Autodesk Inventor part; units mm, degrees
ref_plane "YZ Plane" through (0, 0, 0) normal (1, 0, 0) x (0, 1, 0)
ref_plane "XZ Plane" through (0, 0, 0) normal (0, 1, 0) x (-1, 0, 0)
ref_plane "XY Plane" through (0, 0, 0) normal (0, 0, 1) x (1, 0, 0)
sketch "Sketch1" plane through (0, 0, 0) normal (0, 0, 1) x (1, 0, 0)
  arc A0 (0, 0) -> (0.159434, 1.869277) centre (-11009.945504, 940) ccw construction
  arc A1 (-1.349222, -1.302929) -> (0.159434, 1.869277) centre (-4.822514, 2.29377) ccw
  line L0 (-41.190716, -50.91694) -> (-46.757087, -45.152794) construction
  line L1 (-46.757087, -45.152794) -> (-1.349222, -1.302929)
  arc A2 (0.159434, 1.869277) -> (0, 1880) centre (-11009.945504, 940) ccw
  line L2 (-1.349222, -1.302929) -> (0, 0) construction
  line L3 (0, 0) -> (0, 1880) construction
  line L4 (0, 0) -> (1.875639, 0) construction
  dimension "d148" = 5
  dimension "d153" = 65
  dimension "d165" = 11050
  dimension "d167" = 136
  dimension "d168" = 1880
contour flange "Contour Flange2" sketch "Sketch1" thickness 3 bend radius 5 width 497 along (0, 0, 1) mid plane no both sides no wall seen from (-24.053155, -23.227861, 0) lies toward (0.6946584, -0.7193398, 0) curves L1 A1 A2
bend "Bend2"
corner "Corner2"
sketch "Sketch4" plane through (-1.349222, -1.302929, 497) normal (-0.6946584, 0.7193398, 0) x (0.7193398, 0.6946584, 0)
  line L0 (-81.994451, 7.589283) -> (-81.994451, 144.595466) construction
  line L1 (-81.994451, 144.595466) -> (-67.034181, 144.595466) construction
  line L2 (-67.034181, 144.595466) -> (-67.034181, 7.589283) construction
  line L3 (-67.034181, 7.589283) -> (-81.994451, 7.589283) construction
  point P0 (1.875639, 497)
feature "Mark3" [suppressed]
equation "\"d36\" = Thickness"
equation "\"d37\" = BendReliefWidth"
equation "\"d38\" = BendReliefDepth"
equation "\"d39\" = MinimumRemnant"
equation "\"d40\" = TransitionRadius"
equation "\"d42\" = BendRadius"
equation "\"d44\" = CornerReliefSize"
equation "\"d45\" = GapSize"
equation "\"d46\" = JacobiRadiusSize"
equation "\"BendReliefWidth\" = Thickness"
equation "\"BendReliefDepth\" = 0.5 * Thickness"
equation "\"CornerReliefSize\" = 4 * Thickness"
equation "\"MinimumRemnant\" = 2 * Thickness"
equation "\"GapSize\" = Thickness"
properties part number "MSC 301 sheet left-right board hip" material "Stainless Steel AISI 304"
The model under review builds one solid part; all positions refer to its coordinate system, in mm. Coordinates: 2 decimals unless noted, no trailing zeros. Order: outer loops, then holes, each group sorted by start corner. A loop starts at its lowest first (then second) coordinate and runs counter-clockwise, first axis right, second up. Notation, with made-up numbers: M -15.75,-36 L 6.25,-36 A19 ccw 6.25,-6 Z; hole C 68,7.25 d7. An arc over 180 degrees is marked long. One line per question, with ' | ' between items.
(1) The part is to be moulded in two halves that separate along Y. For faces 1 (the face through (-22.287, -25.693, 245.021)), 2 (the face through (42, 921, 0)), 3 (the face through (43.045, 954.105, 245.021)), 4 (the face through (40.045, 954.101, 245.021)), say which applies: +Y half, -Y half, draft (parallel to the pull), parting line (faces both ways), or undercut.
Geometry results:
face 1: -Y half | face 2: draft | face 3: parting line | face 4: undercut
(2) Insertion check: pin 1 (1.5 mm diameter, centred on x = -25.5, z = 223.5, fed in from +Y); pin 2 (10 mm diameter, centred on x = -36, z = 265.5, fed in from -Y). Each pin has a flat end and moves straight along its axis. Give the tip position at first contact, or say it passes through.
Geometry results:
pin 1: stops at y = -23.9 | pin 2: stops at y = -43.76
(3) Add section A-A, the plane z = 395. Write out the cut boundary in (x, y), then the cut area to 3 significant figures.
Geometry results:
outline: M -46.76,-45.15 L -44.67,-47.31 L 0.73,-3.46 A8 ccw 3.15,1.61 A11053 ccw 2.99,1880.26 L 0,1880 A11050 cw 0.16,1.87 A5 cw -1.35,-1.3 Z | area: 5,850 mm²
(4) Add section C-C, the plane y = 1508. Write out the cut boundary in (x, z).
Geometry results:
outline: M 25.45,0 L 28.45,0 L 28.45,497 L 25.45,497 Z
(5) For probe 1 along Y at (x, z) = (-8, 224); probe 2 along X at (y, z) = (1333, 283); probe 3 along Y at (x, z) = (-4, 301.5), list the stretches that pass through material, from the lowest coordinate up. Write a range as from..to.
Geometry results:
probe 1: y = -11.9..-7.73 | probe 2: x = 33.06..36.07 | probe 3: y = -8.03..-3.86
(6) Add section D-D, the plane y = 842.5. Write out the cut boundary in (x, z), then the cut area to 3 significant figures.
Geometry results:
outline: M 39.62,0 L 42.62,0 L 42.62,497 L 39.62,497 Z | area: 1,490 mm²
